CAD build for the part. Positions are in the model's coordinates, mm. A direction names the side the tool comes from. Coordinates: 2 decimals unless noted, no trailing zeros. Loops run counter-clockwise (first coordinate to the right, second up) from the corner with the lowest first, then second, coordinate; pieces in that order, holes last. Notation, with made-up numbers: M -4,76 L 35,76 A11 ccw 35,88 Z; hole C -31,84.5 d11. An arc over 180 degrees is marked long. Answer as a JSON object with one key per item and string values. Group by question number.
```python
from build123d import *

# Parameters (mm, degrees)
CYLINDER027_R       = 4.1
CYLINDER027_DEPTH   = 24
ARRAY001005_X_COUNT = 2
ARRAY001005_X_PITCH = 90
ARRAY001005_Y_COUNT = 2
ARRAY001005_Y_PITCH = 50
CYLINDER028_R       = 4.5
CYLINDER028_DEPTH   = 10
CYLINDER016_R       = 1.2
CYLINDER016_DEPTH   = 20
ARRAY001006_X_COUNT = 2
ARRAY001006_X_PITCH = 22
ARRAY001006_Y_COUNT = 2
ARRAY001006_Y_PITCH = 22
CYLINDER029_R       = 11.1
CYLINDER029_DEPTH   = 30
CYLINDER036_R       = 2.4
CYLINDER036_DEPTH   = 30
ARRAY001018_Y_COUNT = 2
ARRAY001018_Y_PITCH = 29
CYLINDER037_R       = 23
CYLINDER037_DEPTH   = 30
CYLINDER039_R       = 1.45
CYLINDER039_DEPTH   = 40
ARRAY001020_X_COUNT = 2
ARRAY001020_X_PITCH = 20
ARRAY001021_X_COUNT = 2
ARRAY001021_X_PITCH = 90
CYLINDER040_R       = 1
CYLINDER040_DEPTH   = 10
ARRAY001022_Y_COUNT = 2
ARRAY001022_Y_PITCH = 92
CYLINDER026_R       = 11.2
CYLINDER026_DEPTH   = 10
BOX004_W            = 120
BOX004_H            = 84
BOX004_DEPTH        = 10
BOX019_W            = 30
BOX019_H            = 100
BOX019_DEPTH        = 10


with BuildPart() as rod_hole_array001:
    # Cylinder027 → Cylinder027 (new body)
    with BuildSketch(Plane(origin=(14, 14, 3), x_dir=(1, 0, 0), z_dir=(0, 0, 1))):
        Circle(CYLINDER027_R)
    extrude(amount=CYLINDER027_DEPTH)

    # Array001005 X: rod hole array001 ×2


with BuildPart() as rod_hole_array001_1:
    add(rod_hole_array001.part)
    with Locations(*[(i * ARRAY001005_X_PITCH, 0, 0) for i in range(1, ARRAY001005_X_COUNT)]):
        add(rod_hole_array001.part)

    # Array001005 Y: rod hole array001 ×2


with BuildPart() as rod_hole_array001_2:
    add(rod_hole_array001_1.part)
    with Locations(*[(0, i * ARRAY001005_Y_PITCH, 0) for i in range(1, ARRAY001005_Y_COUNT)]):
        add(rod_hole_array001_1.part)


with BuildPart() as bottom_side_lead_hole:
    # Cylinder028 → Cylinder028 (new body)
    with BuildSketch(Plane(origin=(100, 40, 4), x_dir=(1, 0, 0), z_dir=(0, 0, 1))):
        Circle(CYLINDER028_R)
    extrude(amount=CYLINDER028_DEPTH)


with BuildPart() as lead_holder_hole_array:
    # Cylinder016 → Cylinder016 (new body)
    with BuildSketch(Plane(origin=(-11, -11, 0), x_dir=(1, 0, 0), z_dir=(0, 0, 1))):
        Circle(CYLINDER016_R)
    extrude(amount=CYLINDER016_DEPTH)

    # Array001006 X: lead holder hole array ×2


with BuildPart() as lead_holder_hole_array_1:
    add(lead_holder_hole_array.part)
    with Locations(*[(i * ARRAY001006_X_PITCH, 0, 0) for i in range(1, ARRAY001006_X_COUNT)]):
        add(lead_holder_hole_array.part)

    # Array001006 Y: lead holder hole array ×2


with BuildPart() as lead_holder_hole_array_2:
    add(lead_holder_hole_array_1.part)
    with Locations(*[(0, i * ARRAY001006_Y_PITCH, 0) for i in range(1, ARRAY001006_Y_COUNT)]):
        add(lead_holder_hole_array_1.part)


with BuildPart() as lead_holder_hole_array_3:
    # Array001006 placement: moved
    add(lead_holder_hole_array_2.part.moved(Location((100, 40, -5))))


with BuildPart() as motor_bearing_hole:
    # Cylinder029 → Cylinder029 (new body)
    with BuildSketch(Plane(origin=(49, 40, 0), x_dir=(1, 0, 0), z_dir=(0, 0, 1))):
        Circle(CYLINDER029_R)
    extrude(amount=CYLINDER029_DEPTH)


with BuildPart() as motor_bolt_hole_array:
    # Cylinder036 → Cylinder036 (new body)
    with BuildSketch(Plane.XY):
        Circle(CYLINDER036_R)
    extrude(amount=CYLINDER036_DEPTH)

    # Array001018 Y: motor bolt hole array ×2


with BuildPart() as motor_bolt_hole_array_1:
    add(motor_bolt_hole_array.part)
    with Locations(*[(0, i * ARRAY001018_Y_PITCH, 0) for i in range(1, ARRAY001018_Y_COUNT)]):
        add(motor_bolt_hole_array.part)


with BuildPart() as motor_bolt_hole_array_2:
    # Array001018 placement: moved
    add(motor_bolt_hole_array_1.part.moved(Location((49, 25.5, -6))))


with BuildPart() as motor_body_bottom_hole:
    # Cylinder037 → Cylinder037 (new body)
    with BuildSketch(Plane(origin=(49, 40, 5), x_dir=(1, 0, 0), z_dir=(0, 0, 1))):
        Circle(CYLINDER037_R)
    extrude(amount=CYLINDER037_DEPTH)


with BuildPart() as side_connector_narrow_hole_array_array:
    # Cylinder039 → Cylinder039 (new body)
    with BuildSketch(Plane.XZ):
        Circle(CYLINDER039_R)
    extrude(amount=CYLINDER039_DEPTH)

    # Array001020 X: side connector narrow hole array array ×2


with BuildPart() as side_connector_narrow_hole_array_array_1:
    add(side_connector_narrow_hole_array_array.part)
    with Locations(*[(i * ARRAY001020_X_PITCH, 0, 0) for i in range(1, ARRAY001020_X_COUNT)]):
        add(side_connector_narrow_hole_array_array.part)


with BuildPart() as side_connector_narrow_hole_array_array_2:
    # Array001020 placement: moved
    add(side_connector_narrow_hole_array_array_1.part.moved(Location((5, 0, 5))))

    # Array001021 X: side connector narrow hole array array ×2


with BuildPart() as side_connector_narrow_hole_array_array_3:
    add(side_connector_narrow_hole_array_array_2.part)
    with Locations(*[(i * ARRAY001021_X_PITCH, 0, 0) for i in range(1, ARRAY001021_X_COUNT)]):
        add(side_connector_narrow_hole_array_array_2.part)


with BuildPart() as side_connector_narrow_hole_array_array_4:
    # Array001021 placement: moved
    add(side_connector_narrow_hole_array_array_3.part.moved(Location((0, 27, 0))))


with BuildPart() as body007:
    # Body007 base: copy of side connector narrow hole array array
    add(side_connector_narrow_hole_array_array_4.part)


with BuildPart() as body008:
    # Body008 base: copy of side connector narrow hole array array
    add(side_connector_narrow_hole_array_array_4.part)


with BuildPart() as body008_1:
    # Body008 placement: moved
    add(body008.part.moved(Location((0, 67, 0))))


with BuildPart() as pusher_hole_array:
    # Cylinder040 → Cylinder040 (new body)
    with BuildSketch(Plane(origin=(105, 0, 0), x_dir=(1, 0, 0), z_dir=(0, 0, 1))):
        Circle(CYLINDER040_R)
    extrude(amount=CYLINDER040_DEPTH)

    # Array001022 Y: pusher hole array ×2


with BuildPart() as pusher_hole_array_1:
    add(pusher_hole_array.part)
    with Locations(*[(0, i * ARRAY001022_Y_PITCH, 0) for i in range(1, ARRAY001022_Y_COUNT)]):
        add(pusher_hole_array.part)


with BuildPart() as pusher_hole_array_2:
    # Array001022 placement: moved
    add(pusher_hole_array_1.part.moved(Location((0, -6, 0))))


with BuildPart() as bottom_hole_fusion:
    # Cylinder026 → Cylinder026 (new body)
    with BuildSketch(Plane(origin=(100, 40, -2.5), x_dir=(1, 0, 0), z_dir=(0, 0, 1))):
        Circle(CYLINDER026_R)
    extrude(amount=CYLINDER026_DEPTH)

    # Fusion012: union rod hole array001, bottom side lead hole, lead holder hole array, motor bearing hole, motor bolt hole array, motor body bottom hole, Body007, Body008, pusher hole array
    add(rod_hole_array001_2.part)
    add(bottom_side_lead_hole.part)
    add(lead_holder_hole_array_3.part)
    add(motor_bearing_hole.part)
    add(motor_bolt_hole_array_2.part)
    add(motor_body_bottom_hole.part)
    add(body007.part)
    add(body008_1.part)
    add(pusher_hole_array_2.part)


with BuildPart() as bottom_side_cube:
    # Box004 → Box004 (new body)
    with BuildSketch(Plane(origin=(0, -2, 0), x_dir=(1, 0, 0), z_dir=(0, 0, 1))):
        with Locations((60, 42)):
            Rectangle(BOX004_W, BOX004_H)
    extrude(amount=BOX004_DEPTH)


with BuildPart() as bottom_side_cut:
    # Box019 → Box019 (new body)
    with BuildSketch(Plane(origin=(90, -10, 0), x_dir=(1, 0, 0), z_dir=(0, 0, 1))):
        with Locations((15, 50)):
            Rectangle(BOX019_W, BOX019_H)
    extrude(amount=BOX019_DEPTH)

    # Fusion014: union bottom side cube
    add(bottom_side_cube.part)

    # Cut004: cut bottom hole fusion
    add(bottom_hole_fusion.part, mode=Mode.SUBTRACT)


solid = bottom_side_cut.part
```
Item 1: Slice it at C-C, the plane y = 25.5. Write the cut outline in (x, z).
Item 2: Drill centre lines: L1, parallel to X at y = 14, z = 6.5; L2, parallel to X at y = 81, z = 5; L3, parallel to X at y = 40, z = 6.6. Where is each one in solid material? Low to high. Write a range as from..to.
Item 3: Slice it at B-B, the plane x = 5. Write the cut outline in (y, z).
Item 4: Slice it at A-A, the plane y = 14. Write the cut outline in (x, z), then the cut area to 3 significant figures.
Item 5: Slice it at D-D, the plane x = 91.5. Write the cut outline in (y, z).
Item 6: Pin check, flat tips, straight feed: pin 1 (4 mm diameter, centred on x = 95, z = 5, fed in from +Y); pin 2 (1.4 mm diameter, centred on x = 25.5, z = 4.5, fed in from +Y); pin 3 (1.5 mm diameter, centred on x = 76, z = 7, fed in from -Y); pin 4 (1.9 mm diameter, centred on x = 89, y = 51, fed in from -Z). Stop position of each tip, or through.
Item 7: Tool access for faces 4 (the cylindrical face through (116.339, 8.759, 4.445)), 5 (the flat face through (25, 54, 5)), 6 (the cylindrical face through (99.904, 14.18, 6.451)): list every direction of +Z, -Z, +X, -X, +Y, -Y with a clear straight run to the whole face (end or side of a thin tool).
Item 8: Pull direction Y, two halves, no side cores. Call faces 1 (the flat face through (44, -2, 5)), 2 (the cylindrical face through (88.81, 40.49, 3.7)), 3 (the cylindrical face through (96.339, 72.252, 4.445)): released by +Y, released by -Y, zero draft, split by the parting line, or undercut.
Computed:
{
 "1": {"outline": "M 0,0 L 46.6,0 L 46.6,5 L 31.15,5 L 31.15,10 L 0,10 Z; M 51.4,0 L 120,0 L 120,10 L 66.85,10 L 66.85,5 L 51.4,5 Z; hole C 5,5 d2.9; hole C 25,5 d2.9; hole C 95,5 d2.9; hole C 115,5 d2.9"},
 "2": {"L1": "0..9.9, 18.1..99.9, 108.1..120", "L2": "0..3.55, 6.45..23.55, 26.45..93.55, 96.45..113.55, 116.45..120", "L3": "0..26, 72..88.8, 111.2..120"},
 "3": {"outline": "M -2,0 L 82,0 L 82,3.55 L 54,3.55 L 54,6.45 L 82,6.45 L 82,10 L -2,10 L -2,6.45 L 27,6.45 L 27,3.55 L -2,3.55 Z"},
 "4": {"outline": "M 0,0 L 120,0 L 120,10 L 108.1,10 L 108.1,3 L 99.9,3 L 99.9,10 L 18.1,10 L 18.1,3 L 9.9,3 L 9.9,10 L 0,10 Z; hole C 5,5 d2.9; hole C 25,5 d2.9; hole C 95,5 d2.9; hole C 115,5 d2.9", "area": "1,060 mm2"},
 "5": {"outline": "M -10,0 L 32.71,0 L 32.71,7.5 L 47.29,7.5 L 47.29,0 L 90,0 L 90,10 L -10,10 Z"},
 "6": {"pin 1": "y = 90", "pin 2": "y = 54", "pin 3": "y = -2", "pin 4": "through"},
 "7": {"face 4": "-Y", "face 5": "+Y", "face 6": "+Z"},
 "8": {"face 1": "released by -Y", "face 2": "undercut", "face 3": "zero draft"}
}
